from build123d import *

# Parameters (mm, degrees)
SKETCH1_W           = 47
SKETCH1_H           = 29
SKETCH1_R           = 1.25
SKETCH1_R_2         = 5
BOSS_EXTRUDE1_DEPTH = 4
SKETCH3_W           = 8
SKETCH3_H           = 8
BOSS_EXTRUDE2_DEPTH = 22.5
FILLET1_R           = 1
FILLET2_R           = 5


# Read off the part's stored shape, not the designer's step: Mirror3
with BuildPart() as part:
    # Sketch1 → Boss-Extrude1 (new body)
    with BuildSketch(Plane.XY):
        Rectangle(SKETCH1_W, SKETCH1_H)
        with Locations((7.75, -7.75)):
            Circle(SKETCH1_R, mode=Mode.SUBTRACT)
        with Locations((7.75, 7.75)):
            Circle(SKETCH1_R, mode=Mode.SUBTRACT)
        with Locations((-7.75, 7.75)):
            Circle(SKETCH1_R, mode=Mode.SUBTRACT)
        Circle(SKETCH1_R_2, mode=Mode.SUBTRACT)
        with Locations((-7.75, -7.75)):
            Circle(SKETCH1_R, mode=Mode.SUBTRACT)
    extrude(amount=-BOSS_EXTRUDE1_DEPTH)

    # Sketch3 → Boss-Extrude2 (add)
    with BuildSketch(Plane(origin=(0, 0, -4), x_dir=(-1, 0, 0), z_dir=(0, 0, -1))):
        with Locations((19.5, -10.5)):
            Rectangle(SKETCH3_W, SKETCH3_H)
        with Locations((-19.5, -10.5)):
            Rectangle(SKETCH3_W, SKETCH3_H)
        with Locations((-19.5, 10.5)):
            Rectangle(SKETCH3_W, SKETCH3_H)
        with Locations((19.5, 10.5)):
            Rectangle(SKETCH3_W, SKETCH3_H)
    extrude(amount=BOSS_EXTRUDE2_DEPTH)

    # Fillet1
    fillet1_edges = [part.edges().sort_by_distance(p)[0] for p in [
        (-15.5, -6.5, -15.25),
        (15.5, -6.5, -15.25),
        (15.5, 6.5, -15.25),
        (-15.5, 6.5, -15.25),
        (23.5, -14.5, -13.25),
        (-23.5, -14.5, -13.25),
        (-23.5, 14.5, -13.25),
        (23.5, 14.5, -13.25),
    ]]
    fillet(fillet1_edges, radius=FILLET1_R)

    # Fillet2
    fillet2_edges = [part.edges().sort_by_distance(p)[0] for p in [
        (15.792893219, 6.792893219, -4),
        (-15.792893219, 6.792893219, -4),
        (-15.792893219, -6.792893219, -4),
        (15.792893219, -6.792893219, -4),
        (-20, -6.5, -4),
        (15.5, -11, -4),
        (20, 6.5, -4),
        (-15.5, 11, -4),
        (15.5, 11, -4),
        (-20, 6.5, -4),
        (-15.5, -11, -4),
        (20, -6.5, -4),
    ]]
    fillet(fillet2_edges, radius=FILLET2_R)

    # Mirror3: part across plane


with BuildPart() as part_1:
    add(part.part)
    add(part.part.mirror(Plane.XY.offset(-26.5)))


solid = part_1.part
Check sheet for the modelled part. Datum: model origin and axes. Units: mm. A direction names the side the tool comes from. Give positions to 0.01 mm unless a question says otherwise; leave off trailing zeros. Write each loop counter-clockwise with the first axis right and the second up, starting at its lowest first coordinate (ties: lowest second). Pieces come first, ordered by that corner, then holes. Notation, with made-up numbers: M 46.25,-26 L 76.25,-26 A14 cw 76.25,-21 Z; hole C 44.25,12 d7. An arc over 180 degrees is marked long. Use one line per item in the form item = value.
(1) Section check C-C on x = 7.75. Record the boundary of the cut face in (y, z).
Answer block:
outline = M -14.5,-53 L -9,-53 L -9,-49 L -14.5,-49 Z; M -14.5,-4 L -9,-4 L -9,0 L -14.5,0 Z; M -6.5,-53 L 6.5,-53 L 6.5,-49 L -6.5,-49 Z; M -6.5,-4 L 6.5,-4 L 6.5,0 L -6.5,0 Z; M 9,-53 L 14.5,-53 L 14.5,-49 L 9,-49 Z; M 9,-4 L 14.5,-4 L 14.5,0 L 9,0 Z
(2) Draft check along X on faces 1 (the flat face through (20, -6.5, -27)), 2 (the cylindrical face through (6.5, -7.7, -51)), 3 (the flat face through (-23.5, 9, -27)). Enter one of: pulls with the +X half, pulls with the -X half, needs draft (parallel to the pull), parting line crosses it, or undercut.
Answer block:
face_1 = needs draft
face_2 = undercut
face_3 = pulls with the -X half
(3) Section check D-D on z = -16. Record the boundary of the cut face in (x, y), plus the area to 3 significant figures.
Answer block:
outline = M -23.5,-13.5 A1 ccw -22.5,-14.5 L -15.5,-14.5 L -15.5,-7.5 A1 ccw -16.5,-6.5 L -23.5,-6.5 Z; M -23.5,6.5 L -16.5,6.5 A1 ccw -15.5,7.5 L -15.5,14.5 L -22.5,14.5 A1 ccw -23.5,13.5 Z; M 15.5,-14.5 L 22.5,-14.5 A1 ccw 23.5,-13.5 L 23.5,-6.5 L 16.5,-6.5 A1 ccw 15.5,-7.5 Z; M 15.5,7.5 A1 ccw 16.5,6.5 L 23.5,6.5 L 23.5,13.5 A1 ccw 22.5,14.5 L 15.5,14.5 Z
area = 254 mm2
(4) Section check B-B on y = 0. Record the boundary of the cut face in (x, z).
Answer block:
outline = M -23.5,-53 L -5,-53 L -5,-49 L -23.5,-49 Z; M -23.5,-4 L -5,-4 L -5,0 L -23.5,0 Z; M 5,-53 L 23.5,-53 L 23.5,-49 L 5,-49 Z; M 5,-4 L 23.5,-4 L 23.5,0 L 5,0 Z
(5) Material ranges on line 1 along Y through (x, z) = (0, -51.1); line 2 along Z through (x, y) = (12.5, -0.25); line 3 along Y through (x, z) = (-7.75, -50.7), recorded low to high.
Answer block:
line_1 = -14.5 to -5, 5 to 14.5
line_2 = -53 to -49, -4 to 0
line_3 = -14.5 to -9, -6.5 to 6.5, 9 to 14.5
(6) Depth check by flat-ended pin: P1, Ø2, axis at x = -7.75, y = -7.75, coming from the -Z side. Enter the tip coordinate at first touch or a pass-through.
Answer block:
P1 = through
(7) Section check A-A on x = 0. Record the boundary of the cut face in (y, z).
Answer block:
outline = M -14.5,-53 L -5,-53 L -5,-49 L -14.5,-49 Z; M -14.5,-4 L -5,-4 L -5,0 L -14.5,0 Z; M 5,-53 L 14.5,-53 L 14.5,-49 L 5,-49 Z; M 5,-4 L 14.5,-4 L 14.5,0 L 5,0 Z
(8) Tool access check on faces 4 (the cylindrical face through (14, 10.95, -47.57)), 5 (the flat face through (-6, 0, -53)), 6 (the cylindrical face through (-20.05, -5, -5.43)). Record the directions out of +Z, -Z, +X, -X, +Y, -Y that give a thin tool (end or side, any length) a straight path to the whole face; none if there is none.
Answer block:
face_4 = +Y, -Y
face_5 = -Z, +X, -X, +Y, -Y
face_6 = +X, -X
